Geometry check sheet. Reference: the model listing, model coordinates, mm. Face numbers are marked on the shaded views. A direction names the side the tool comes from. Give positions to 0.01 mm unless a question says otherwise; leave off trailing zeros. Loops run counter-clockwise (first coordinate to the right, second up) from the corner with the lowest first, then second, coordinate; pieces in that order, holes last. Notation, with made-up numbers: (61, -25) -> (92, -25) arc R14 ccw to (92, -3) -> close; hole circle Ø10 at (-1.5, 63). An arc over 180 degrees is marked (long way). One line per item, written item: value. Start each with the question number.
(1) Tool access check on the marked faces 1, 2 and 3. Record the directions out of +Z, -Z, +X, -X, +Y, -Y that give a thin tool (end or side, any length) a straight path to the whole face; none if there is none.
(2) Sectioned sample at C-C, the plane y = -104.5. Record the cut outline in (x, z), then the cut area to 3 significant figures.
(3) Gauge pin test, flat ends, axial feed: pin 1 Ø2.5 at (x, z) = (-57, -3.5) entering from +Y; pin 2 Ø4 at (x, y) = (-56.5, -91.5) entering from +Z; pin 3 Ø2 at (x, y) = (-53.5, -67.5) entering from -Z. Record the tip position at first contact, or that the pin passes through.
(4) Sectioned sample at A-A, the plane z = -40.07. Record the cut outline in (x, y), then the cut area to 3 significant figures.
(5) Sectioned sample at B-B, the plane x = -55.5. Record the cut outline in (y, z), then the cut area to 3 significant figures.
(6) Scan lines: line 1 along Y through (x, z) = (-54.25, -90.07); line 2 along Z through (x, y) = (-57.75, -85); line 3 along Z through (x, y) = (-54.5, -97). Record each from-to range of solid material in increasing order. Write a range as from..to.
from build123d import *

# Parameters (mm, degrees)
SKETCH1_W           = 8
SKETCH1_H           = 15
BOSS_EXTRUDE1_DEPTH = 10
BOSS_EXTRUDE2_DEPTH = 110.14
FILLET1_R           = 10
SKETCH4_R           = 2.5
CUT_EXTRUDE1_DEPTH  = 10


with BuildPart() as part:
    # Sketch1 → Boss-Extrude1 (new body)
    with BuildSketch(Plane.XY):
        with Locations((-55, -78)):
            Rectangle(SKETCH1_W, SKETCH1_H)
    boss_extrude1 = extrude(amount=-BOSS_EXTRUDE1_DEPTH)

    # Sketch2 → Boss-Extrude2 (add)
    with BuildSketch(Plane(origin=(0, 0, -10), x_dir=(-1, 0, 0), z_dir=(0, 0, -1))):
        Polygon((51, -62.565581077), (59, -62.565581077), (59, -92.565581077), (59, -107.565581077), (51, -107.565581077), (51, -92.565581077), align=None)
    extrude(amount=BOSS_EXTRUDE2_DEPTH)

    # Fillet1
    fillet1_edges = [part.edges().sort_by_distance(p)[0] for p in [
        (-55, -107.565581077, -120.14),
        (-55, -107.565581077, -10),
    ]]
    fillet(fillet1_edges, radius=FILLET1_R)

    # Mirror1: Boss-Extrude1 across plane
    add(boss_extrude1.mirror(Plane.XY.offset(-65.07)))

    # Sketch4 → Cut-Extrude1 (cut)
    with BuildSketch(Plane(origin=(-51, 0, 0), x_dir=(0, 0, -1), z_dir=(1, 0, 0))):
        with Locations((40.07, -85.065581077)):
            Circle(SKETCH4_R)
        with Locations(Location((90.07, -85.065581077, 0), (0, 0, 180))):
            Circle(SKETCH4_R)
    extrude(amount=-CUT_EXTRUDE1_DEPTH, mode=Mode.SUBTRACT)


solid = part.part
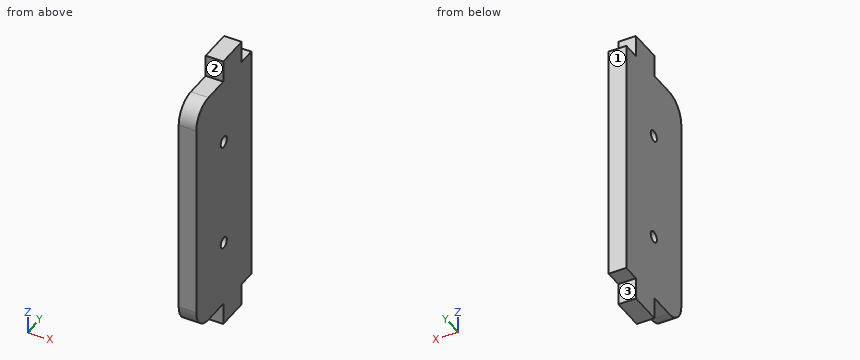
Calculated:
1. face 1: +Z, -Z, +X, -X, +Y
1. face 2: +Z, +X, -X, -Y
1. face 3: -Z, +X, -X, +Y
2. outline: (-59, -117.35) -> (-51, -117.35) -> (-51, -12.79) -> (-59, -12.79) -> close
2. area: 836 mm2
3. pin 1: stops at y = -70.5
3. pin 2: stops at z = -10
3. pin 3: stops at z = -120.14
4. outline: (-59, -107.57) -> (-51, -107.57) -> (-51, -87.57) -> (-59, -87.57) -> close; (-59, -82.57) -> (-51, -82.57) -> (-51, -62.57) -> (-59, -62.57) -> close
4. area: 320 mm2
5. outline: (-107.57, -110.14) arc R10 ccw to (-97.57, -120.14) -> (-85.5, -120.14) -> (-85.5, -130.14) -> (-70.5, -130.14) -> (-70.5, -120.14) -> (-62.57, -120.14) -> (-62.57, -10) -> (-70.5, -10) -> (-70.5, 0) -> (-85.5, 0) -> (-85.5, -10) -> (-97.57, -10) arc R10 ccw to (-107.57, -20) -> close; hole circle Ø5 at (-85.07, -90.07); hole circle Ø5 at (-85.07, -40.07)
5. area: 5,170 mm2
6. line 1: y = -107.57..-87.57, -82.57..-62.57
6. line 2: z = -130.14..-92.57, -87.57..-42.57, -37.57..0
6. line 3: z = -120.14..-10
